```python
from build123d import *

# Parameters (mm, degrees)
F1_DEPTH = 70
F2_SIZE  = 10
F3_R     = 5
F4_R     = 21.491967
F5_DEPTH = 39.1
F6_R     = 26.594603
F7_DEPTH = 25


with BuildPart() as f1:
    # F0 (on Front) → F1 (new body)
    with BuildSketch(Plane.XZ):
        Polygon((23.009436, 48.425878), (-34.368057, 48.425878), (-54.164968, 30.633396), (-54.164968, -28.757341), (-41.078873, -51.574122), (27.371468, -51.574122), (45.835032, -33.119373), (45.835032, 34.995425), align=None)
    extrude(amount=F1_DEPTH)

    # F2
    f2_edges = [f1.edges().sort_by_distance(p)[0] for p in [
        (-5.67931, 0, 48.425878),
        (-44.266513, 0, 39.529637),
        (-54.164968, 0, 0.938027),
        (-47.621921, 0, -40.165732),
        (-6.853702, 0, -51.574122),
        (36.60325, 0, -42.346748),
        (45.835032, 0, 0.938026),
        (34.422234, 0, 41.710652),
    ]]
    chamfer(f2_edges, length=F2_SIZE)

    # F3
    f3_edges = [f1.edges().sort_by_distance(p)[0] for p in [
        (-5.67931, -70, 48.425878),
        (-44.266513, -70, 39.529637),
        (-54.164968, -70, 0.938027),
        (-47.621921, -70, -40.165732),
        (-6.853702, -70, -51.574122),
        (36.60325, -70, -42.346748),
        (45.835032, -70, 0.938026),
        (34.422234, -70, 41.710652),
    ]]
    fillet(f3_edges, radius=F3_R)

    # F4 (on face) → F5 (join)
    with BuildSketch(Plane(origin=(0, 0, 0), x_dir=(-1, 0, 0), z_dir=(0, 1, 0))):
        Circle(F4_R)
    extrude(amount=-F5_DEPTH)

    # F6 (on face) → F7 (cut)
    with BuildSketch(Plane.XZ.offset(70)):
        with Locations((-9.82369, -4.344146)):
            Circle(F6_R)
    extrude(amount=-F7_DEPTH, mode=Mode.SUBTRACT)


solid = f1.part
```
Input: part model. Units: mm. Frame: model coordinates. A direction names the side the tool comes from. Coordinates: 2 decimals unless noted, no trailing zeros. Loops run counter-clockwise (first coordinate to the right, second up) from the corner with the lowest first, then second, coordinate; pieces in that order, holes last. Notation, with made-up numbers: M 62,-13.5 L 79,-13.5 A17 ccw 79,-6.5 Z; hole C 26.25,52 d2. An arc over 180 degrees is marked long. Use a Markdown table: item, result. Add a question column.
1) Pin query (flat end, axial travel): P1, Ø10, axis at x = -10.5, z = -20, coming from the -Y side. Return the tip coordinate at first contact, or that it passes through.
2) Section B-B, the plane z = 13. Return the cut outline in (x, y).
3) Draft query along Z for faces 3 (the flat face through (-10, -45, -4)), 4 (the flat face through (36.47, -37.11, -42.48)), 5 (the cylindrical face through (44.331, -68.574, 1.415)). Return one class per face: +Z half, -Z half, draft (parallel to the pull), parting line (faces both ways), or undercut.
4) Section D-D, the plane y = -5. Return the cut outline in (x, z), plus the area to 3 significant figures.
5) Section A-A, the plane y = -21.5. Return the cut outline in (x, z), plus the area to 3 significant figures.
6) Line query: L1, parallel to Y at x = 0, z = 20; L2, parallel to X at y = -60.5, z = -8.5; L3, parallel to X at y = -4, z = 41. Output: solid intervals per line, ascending. Write a range as from..to.
7) Set-up query: faces 1 (the cylindrical face through (-30.928, -57.675, -20.527)), 2 (the flat face through (45.835, -37, 0)). Return all of +Z, -Z, +X, -X, +Y, -Y with unobstructed straight access to the full face (end or side cutting, diameter ignored); none if empty.
8) Section C-C, the plane x = -15.5. Return the cut outline in (y, z), plus the area to 3 significant figures.
Answer below:
| question | item | result |
|---|---|---|
| 1 | P1 | y = -45 |
| 2 | outline | M -54.16,-65 A5 ccw -49.16,-70 L -29.98,-70 L -29.98,-45 L 10.34,-45 L 10.34,-70 L 40.84,-70 A5 ccw 45.84,-65 L 45.84,-10 L 35.84,0 L -44.16,0 L -54.16,-10 Z |
| 3 | face 3 | undercut |
| 3 | face 4 | -Z half |
| 3 | face 5 | draft |
| 4 | outline | M -49.16,-27.43 L -38.18,-46.57 L 25.3,-46.57 L 40.84,-31.05 L 40.84,32.14 L 21.65,43.43 L -32.45,43.43 L -49.16,28.4 Z |
| 4 | area | 7,640 mm2 |
| 5 | outline | M -54.16,-28.76 L -41.08,-51.57 L 27.37,-51.57 L 45.84,-33.12 L 45.84,35 L 23.01,48.43 L -34.37,48.43 L -54.16,30.63 Z |
| 5 | area | 9,350 mm2 |
| 6 | L1 | -45..0 |
| 6 | L2 | -54.16..-36.09, 16.44..45.84 |
| 6 | L3 | -33.65..23.8 |
| 7 | face 1 | -Y |
| 7 | face 2 | +Z, -Z, +X, +Y, -Y |
| 8 | outline | M -70,-46.57 A5 ccw -65,-51.57 L -10,-51.57 L 0,-41.57 L 0,38.43 L -10,48.43 L -65,48.43 A5 ccw -70,43.43 L -70,21.64 L -45,21.64 L -45,-30.33 L -70,-30.33 Z |
| 8 | area | 5,590 mm2 |
